from build123d import *

# Parameters (mm, degrees)
BOX006_W        = 88.9
BOX006_H        = 88.9
BOX006_DEPTH    = 2438.4
SKETCH003_W     = 38.1
SKETCH003_H     = 88.9
POCKET003_DEPTH = 88.9010000032
POCKET008_DEPTH = 88.901
POCKET011_DEPTH = 38.1
SKETCH019_W     = 38.1
SKETCH019_H     = 101.6
POCKET016_DEPTH = 88.901


with BuildPart() as part:
    # Box006 → Box006 (new body)
    with BuildSketch(Plane(origin=(1435.1, 1435.1, 0), x_dir=(1, 0, 0), z_dir=(0, 0, 1))):
        with Locations((44.45, 44.45)):
            Rectangle(BOX006_W, BOX006_H)
    extrude(amount=BOX006_DEPTH)

    # Sketch003 → Pocket003 (cut, through all)
    with BuildSketch(Plane(origin=(1435.1, 1435.1, 0), x_dir=(1, 0, 0), z_dir=(0, -1, 0))):
        with Locations((69.85, 501.65)):
            Rectangle(SKETCH003_W, SKETCH003_H)
    extrude(amount=-POCKET003_DEPTH, mode=Mode.SUBTRACT)

    # Sketch009 → Pocket008 (cut, through all)
    with BuildSketch(Plane(origin=(1524, 1435.1, 0), x_dir=(0, 1, 0), z_dir=(1, 0, 0))):
        Polygon((88.9, 2221.9412), (88.9, 2438.4), (0, 2438.4), (0, 2189.5842461737), align=None)
    extrude(amount=-POCKET008_DEPTH, mode=Mode.SUBTRACT)

    # Sketch012 → Pocket011 (cut)
    with BuildSketch(Plane(origin=(1524, 1435.1, 0), x_dir=(0, 1, 0), z_dir=(1, 0, 0))):
        Polygon((0, 2189.5842461737), (0, 2049.8842461737), (88.9, 2082.2412), (88.9, 2221.9412), align=None)
    extrude(amount=-POCKET011_DEPTH, mode=Mode.SUBTRACT)

    # Sketch019 → Pocket016 (cut, through all)
    with BuildSketch(Plane(origin=(1435.1, 1435.1, 0), x_dir=(0, -1, 0), z_dir=(-1, 0, 0))):
        with Locations((-69.85, 2171.7)):
            Rectangle(SKETCH019_W, SKETCH019_H)
    extrude(amount=-POCKET016_DEPTH, mode=Mode.SUBTRACT)


solid = part.part
Input: part model. Units: mm. Frame: model coordinates. A direction names the side the tool comes from. Give positions to 0.01 mm unless a question says otherwise; leave off trailing zeros. Order: outer loops, then holes, each group sorted by start corner. A loop starts at its lowest first (then second) coordinate and runs counter-clockwise, first axis right, second up.
Q1. Set-up query: faces 5 (the flat face through (1505.217, 1478.928, 2065.836)), 6 (the flat face through (1460, 1485.9, 2164)), 7 (the flat face through (1505, 1479, 546.1)). Return all of +Z, -Z, +X, -X, +Y, -Y with unobstructed straight access to the full face (end or side cutting, diameter ignored); none if empty.
Checked values:
face 5: +Z, +X, -Y
face 6: +Z, +X, -X, +Y
face 7: +X, +Y, -Y
Q2. Section A-A on x = 1508.5. Output: boundary loops of the cut face in (y, z).
Checked values:
outline: (1435.1, 0) - (1524, 0) - (1524, 457.2) - (1435.1, 457.2) - close; (1435.1, 546.1) - (1524, 546.1) - (1524, 2082.24) - (1435.1, 2049.88) - close
Q3. Draft query along Z for faces 1 (the flat face through (1505, 1479, 457.2)), 2 (the flat face through (1479, 1435.1, 1079)), 3 (the flat face through (1460.86, 1460.14, 2198.7)), 4 (the flat face through (1485.9, 1479, 501)). Return one class per face: +Z half, -Z half, draft (parallel to the pull), parting line (faces both ways), or undercut.
Checked values:
face 1: undercut
face 2: draft
face 3: +Z half
face 4: undercut
Q4. Ray query, probe 1 along Z at (x, y) = (1450, 1492); probe 2 along Z at (x, y) = (1488, 1457.5); probe 3 along Z at (x, y) = (1512.5, 1511.5). Return the intervals inside material, ascending.
Checked values:
probe 1: z = 0 to 2120.9
probe 2: z = 0 to 457.2, 546.1 to 2058.04
probe 3: z = 0 to 457.2, 546.1 to 2077.69
Q5. Section B-B on y = 1461. Output: boundary loops of the cut face in (x, z), and give its area (3 significant figures).
Checked values:
outline: (1435.1, 0) - (1524, 0) - (1524, 457.2) - (1485.9, 457.2) - (1485.9, 546.1) - (1524, 546.1) - (1524, 2059.31) - (1485.9, 2059.31) - (1485.9, 2199.01) - (1435.1, 2199.01) - close
area: 187,000 mm2
Q6. Contact query for flat-ended pins moving along their axis: pin 1 Ø12 at (x, y) = (1514, 1472) entering from +Z; pin 2 Ø15 at (x, z) = (1455, 2158.5) entering from +Y; pin 3 Ø12 at (x, y) = (1450, 1514) entering from +Z. Output: stop coordinate, or through.
Checked values:
pin 1: stops at z = 2065.5
pin 2: stops at y = 1485.9
pin 3: stops at z = 2120.9
